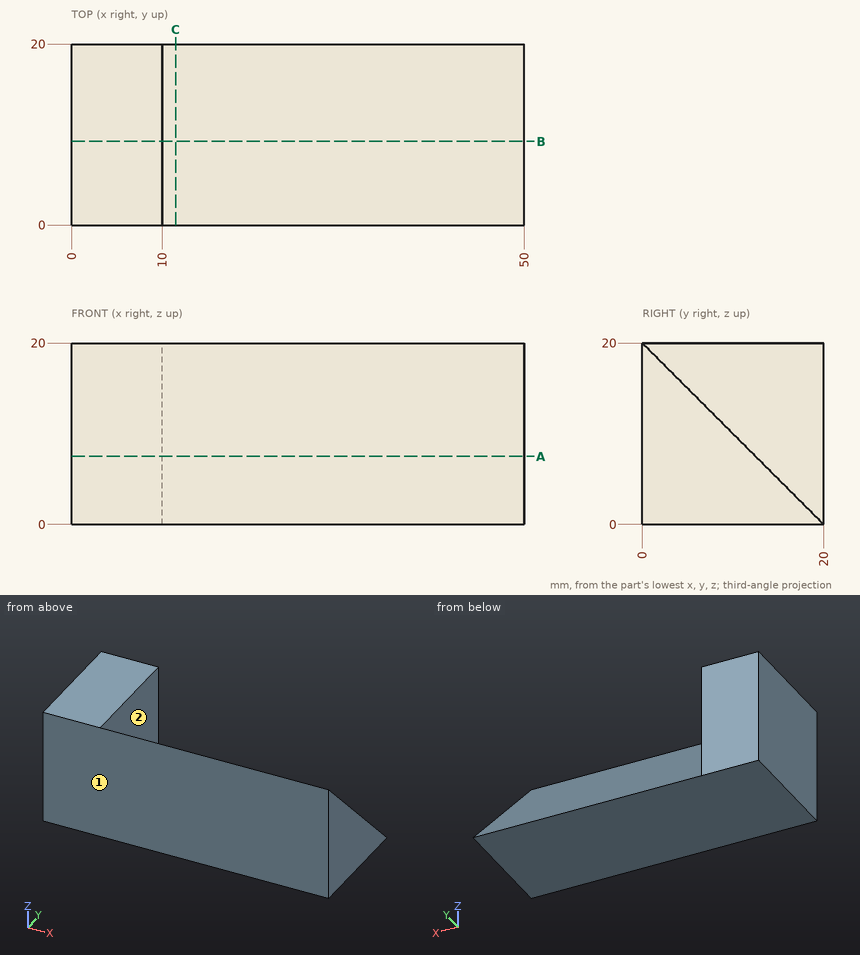
Geometry check sheet. Reference: drawing and pictorial views, mm from the part's lowest x, y, z. A direction names the side the tool comes from. Give positions to 0.01 mm unless a question says otherwise; leave off trailing zeros. Loops run counter-clockwise (first coordinate to the right, second up) from the corner with the lowest first, then second, coordinate; pieces in that order, holes last. Notation, with made-up numbers: (28, -12) - (44, -12) arc R10 cw to (44, 2) - close; hole circle Ø2 at (78.5, 5.25). An arc over 180 degrees is marked (long way). Use CSV: the item, a comma, the result in double quotes. Start each with the question number.
Q1. Scan lines: probe 1 along X at (y, z) = (16.5, 13.5); probe 2 along Y at (x, z) = (35.5, 8). Record each from-to range of solid material in increasing order. Write a range as from..to.
Q2. Section check B-B, the plane y = 9.25. Record the cut outline in (x, z).
Q3. Access from +Z, -Z, +X, -X, +Y, -Y to the whole of each face (thin tool, end or side, straight path). Record for the marked faces 1 and 2.
Q4. Section check C-C, the plane x = 11.5. Record the cut outline in (y, z).
Q5. Go/stop test with flat-tipped pins: pin 1 Ø4 at (x, z) = (28, 15) entering from +Y; pin 2 Ø10 at (x, y) = (25.5, 8.5) entering from +Z. Record where each tip stops, or that it passes through.
Q6. Section check A-A, the plane z = 7.5. Record the cut outline in (x, y).
Findings below:
1,probe 1,"x = 0..10"
1,probe 2,"y = 0..12"
2,outline,"(0, 0) - (50, 0) - (50, 10.75) - (10, 10.75) - (10, 20) - (0, 20) - close"
3,face 1,"+Z, -Z, +X, -X, -Y"
3,face 2,"+Z, +X, +Y"
4,outline,"(0, 0) - (20, 0) - (0, 20) - close"
5,pin 1,"stops at y = 7"
5,pin 2,"stops at z = 16.5"
6,outline,"(0, 0) - (50, 0) - (50, 12.5) - (10, 12.5) - (10, 20) - (0, 20) - close"
